Drawing for the job (mm, zero at the part's lowest x, y, z). A direction names the side the tool comes from. Round coordinates to 2 decimals unless told otherwise and drop trailing zeros. Write each loop counter-clockwise with the first axis right and the second up, starting at its lowest first coordinate (ties: lowest second). Pieces come first, ordered by that corner, then holes.
Item 1: Band-saw the part on A-A, the plane x = 15.5. Write the cut outline in (y, z).
Item 2: Mould opens along Y. For the marked faces 3, 4 and 5 say: +Y half, -Y half, draft (parallel to the pull), parting line (faces both ways), or undercut.
Item 3: Band-saw the part on B-B, the plane y = 14. Write the cut outline in (x, z) (1 decimal).
Item 4: Band-saw the part on D-D, the plane y = 18. Write the cut outline in (x, z) (1 decimal), then the cut area to 3 significant figures.
Item 5: Band-saw the part on C-C, the plane z = 10.5. Write the cut outline in (x, y) (1 decimal).
Item 6: Wall check: probe 1 along Y at (x, z) = (14, 4.25); probe 2 along Z at (x, y) = (11.5, 22.5); probe 3 along Y at (x, z) = (16.25, 5.25) (1 decimal). Give the ranges that are in metal, low to high.
Item 7: Drop flat-ended pins along their axis: pin 1 Ø1 at (y, z) = (20, 3.5) entering from +X; pin 2 Ø4 at (x, y) = (13.86, 12) entering from +Z; pin 3 Ø2 at (y, z) = (3.5, 10) entering from -X; pin 4 Ø3 at (x, z) = (4.5, 11.5) entering from -Y. Give the stop position or say it passes through.
Item 8: 3-axis set-ups, long thin cutter, end or side, ignore diameter. For the marked faces 1 and 2: which of +Z, -Z, +X, -X, +Y, -Y reach the whole face in a straight line?
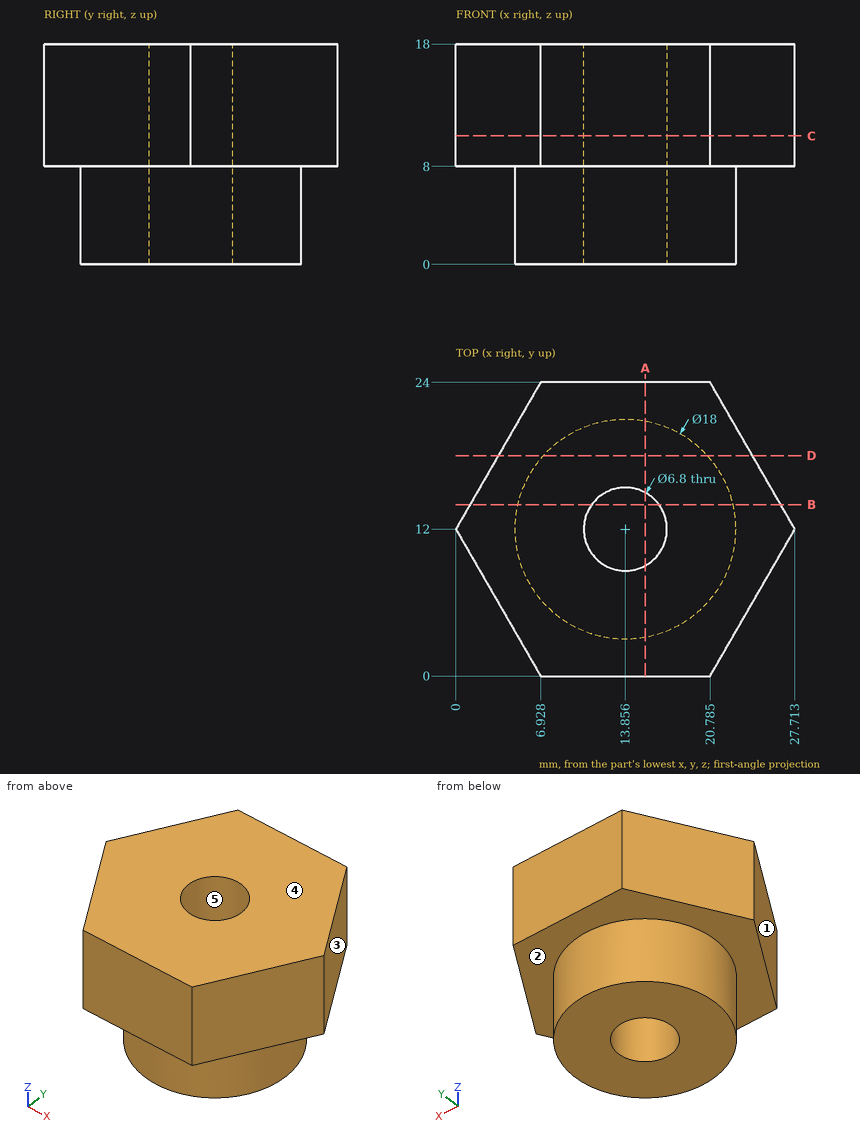
Results:
1. outline: (0, 8) - (3.15, 8) - (3.15, 0) - (9.02, 0) - (9.02, 18) - (0, 18) - close; (14.98, 0) - (20.85, 0) - (20.85, 8) - (24, 8) - (24, 18) - (14.98, 18) - close
2. face 3: +Y half
2. face 4: draft
2. face 5: undercut
3. outline: (1.2, 8) - (5.1, 8) - (5.1, 0) - (11.1, 0) - (11.1, 18) - (1.2, 18) - close; (16.6, 0) - (22.6, 0) - (22.6, 8) - (26.6, 8) - (26.6, 18) - (16.6, 18) - close
4. outline: (3.5, 8) - (7.1, 8) - (7.1, 0) - (20.6, 0) - (20.6, 8) - (24.2, 8) - (24.2, 18) - (3.5, 18) - close
4. area: 315 mm2
5. outline: (0, 12) - (6.9, 0) - (20.8, 0) - (27.7, 12) - (20.8, 24) - (6.9, 24) - close; hole circle Ø6.8 at (13.9, 12)
6. probe 1: y = 3 to 8.6, 15.4 to 21
6. probe 2: z = 8 to 18
6. probe 3: y = 3.3 to 9.6, 14.4 to 20.7
7. pin 1: stops at x = 18.83
7. pin 2: passes through
7. pin 3: stops at x = 4.33
7. pin 4: stops at y = 1.61
8. face 1: +Z, -Z, -X, -Y
8. face 2: -Z
